from build123d import *

# Parameters (mm, degrees)
SKETCH_1_R          = 3
EXTRUDE_1_DEPTH     = 3
EXTRUDE_2_DEPTH     = 3
SKETCH_3_R          = 2.75
EXTRUDE_3_DEPTH     = 1
SKETCH_4_R          = 4
EXTRUDE_4_DEPTH     = 1
SKETCH_5_R          = 2.5
CUT_EXTRUDE_1_DEPTH = 10.797958971


with BuildPart() as part:
    # 草图1 → 凸台-拉伸1 (new body)
    with BuildSketch(Plane(origin=(0, 0, 0), x_dir=(0, 0, -1), z_dir=(1, 0, 0))):
        Circle(SKETCH_1_R)
    extrude(amount=EXTRUDE_1_DEPTH)

    # 草图2 → 凸台-拉伸2 (add)
    with BuildSketch(Plane(origin=(3, 0, 0), x_dir=(0, 0, -1), z_dir=(1, 0, 0))):
        Polygon((3.238836652, -1.228794996), (2.683586009, 2.190517321), (-0.555250643, 3.419312317), (-3.238836652, 1.228794996), (-2.683586009, -2.190517321), (0.555250643, -3.419312317), align=None)
    extrude(amount=EXTRUDE_2_DEPTH)

    # 草图3 → 凸台-拉伸3 (add)
    with BuildSketch(Plane(origin=(6, 0, 0), x_dir=(0, 0, -1), z_dir=(1, 0, 0))):
        Circle(SKETCH_3_R)
    extrude(amount=EXTRUDE_3_DEPTH)

    # 草图4 → 凸台-拉伸4 (add)
    with BuildSketch(Plane(origin=(7, 0, 0), x_dir=(0, 0, -1), z_dir=(1, 0, 0))):
        Circle(SKETCH_4_R)
    extrude(amount=EXTRUDE_4_DEPTH)

    # 草图5 → 切除-拉伸1 (cut, through all)
    with BuildSketch(Plane.ZY):
        Circle(SKETCH_5_R)
    extrude(amount=-CUT_EXTRUDE_1_DEPTH, mode=Mode.SUBTRACT)


solid = part.part
Source: CAD feature listing. Evaluate the final solid. Frame: model axes, mm. A direction names the side the tool comes from. Round coordinates to 2 decimals unless told otherwise and drop trailing zeros. Loops run counter-clockwise (first coordinate to the right, second up) from the corner with the lowest first, then second, coordinate; pieces in that order, holes last.
Q1. Section A-A, the plane x = 3.5. Return loops of the section in (y, z), plus the area to 3 significant figures.
Q2. Access query for faces 1 (the face through (3, 2, -2.5)), 2 (the face through (4.479, -0.457, 2.965)), 3 (the face through (7, 1, -3)), 4 (the face through (4.48, 2.34, 1.88)), 5 (the face through (7.493, -3.905, 0.867)). Directions: +Z, -Z, +X, -X, +Y, -Y. A direction counts if a zero-diameter tool reaches every point of the face in a straight line with its end or side. Return the directions, or none.
Q3. Ray query, line 1 (X direction, y = -1, z = -2.75); line 2 (Y direction, x = 2.75, z = 0); line 3 (X direction, y = -1, z = -3). Return the intervals inside material, ascending.
Q4. First-contact query: P1, Ø2, axis at x = 2.5, z = -0.5, coming from the +Y side; P2, Ø3, axis at x = 1.5, z = -1.5, coming from the +Y side; P3, Ø1, axis at x = 3.5, y = 0, coming from the -Z side. Flat tips, straight axial feed; report the tip coordinate or a pass-through.
Q5. Section D-D, the plane y = 3.25. Return loops of the section in (x, z).
Q6. Section B-B, the plane z = 0. Return loops of the section in (x, y), plus the area to 3 significant figures.
Q7. Mould query, pull axis Z, two halves, no side actions, for faces 6 (the face through (4.48, -2.34, -1.88)), 7 (the face through (3.94, -2.44, -0.54)), 8 (the face through (6.493, -2.685, 0.596)), 9 (the face through (0, 2, 2)). Classes: pulls with the +Z half, pulls with the -Z half, needs draft (parallel to the pull), parting line crosses it, or undercut.
Q8. Section C-C, the plane y = 1. Return loops of the section in (x, z), plus the area to 3 significant figures.
Solutions:
1. outline: (-3.42, -0.56) - (-1.23, -3.24) - (2.19, -2.68) - (3.42, 0.56) - (1.23, 3.24) - (-2.19, 2.68) - close; hole circle Ø5 at (0, 0)
1. area: 11.5 mm2
2. face 1: -Z, -X, +Y
2. face 2: +Z, -X, -Y
2. face 3: none
2. face 4: +Z, -X, +Y
2. face 5: +X, -X
3. line 1: x = 0 to 6, 7 to 8
3. line 2: y = -3 to -2.5, 2.5 to 3
3. line 3: x = 3 to 6, 7 to 8
4. P1: stops at y = 3.35
4. P2: stops at y = 3
4. P3: stops at z = -3.12
5. outline: (3, 0.11) - (6, 0.11) - (6, 0.76) - (3, 0.76) - close; (7, -2.33) - (8, -2.33) - (8, 2.33) - (7, 2.33) - close
6. outline: (0, -3) - (3, -3) - (3, -3.21) - (6, -3.21) - (6, -2.75) - (7, -2.75) - (7, -4) - (8, -4) - (8, -2.5) - (0, -2.5) - close; (0, 2.5) - (8, 2.5) - (8, 4) - (7, 4) - (7, 2.75) - (6, 2.75) - (6, 3.21) - (3, 3.21) - (3, 3) - (0, 3) - close
6. area: 10.8 mm2
7. face 6: pulls with the -Z half
7. face 7: undercut
7. face 8: parting line crosses it
7. face 9: needs draft
8. outline: (0, -2.83) - (3, -2.83) - (3, -2.88) - (6, -2.88) - (6, -2.56) - (7, -2.56) - (7, -3.87) - (8, -3.87) - (8, -2.29) - (0, -2.29) - close; (0, 2.29) - (8, 2.29) - (8, 3.87) - (7, 3.87) - (7, 2.56) - (6, 2.56) - (6, 3.2) - (3, 3.2) - (3, 2.83) - (0, 2.83) - close
8. area: 11.4 mm2
